```python
from build123d import *

# Parameters (mm, degrees)
F0_W     = 20
F0_H     = 20
F0_R     = 1.75
F0_R_2   = 1.1
F1_DEPTH = 3
F2_DEPTH = 1.4
F0_W_2   = 7.5
F3_DEPTH = 15
F4_DEPTH = 3
F5_W     = 3.5
F5_H     = 7.2
F6_DEPTH = 10
F7_R     = 2
F8_DEPTH = 25
F9_DEPTH = 7.5


with BuildPart() as f1:
    # F0 (on Right) → F1 (new body)
    with BuildSketch(Plane.YZ):
        Rectangle(F0_W, F0_H)
        with Locations((-5, -5)):
            Circle(F0_R, mode=Mode.SUBTRACT)
        with Locations((5, -5)):
            Circle(F0_R, mode=Mode.SUBTRACT)
        with Locations((-5, 5)):
            Circle(F0_R, mode=Mode.SUBTRACT)
        with Locations((5, 5)):
            Circle(F0_R, mode=Mode.SUBTRACT)
        with Locations((-5, 5)):
            Circle(F0_R)
        with Locations((-5, 5)):
            Circle(F0_R_2, mode=Mode.SUBTRACT)
        with Locations((5, 5)):
            Circle(F0_R)
        with Locations((5, 5)):
            Circle(F0_R_2, mode=Mode.SUBTRACT)
        with Locations((5, -5)):
            Circle(F0_R)
        with Locations((5, -5)):
            Circle(F0_R_2, mode=Mode.SUBTRACT)
        with Locations((-5, -5)):
            Circle(F0_R)
        with Locations((-5, -5)):
            Circle(F0_R_2, mode=Mode.SUBTRACT)
    extrude(amount=-F1_DEPTH)

    # F0 (on Right) → F2 (cut)
    with BuildSketch(Plane.YZ):
        with Locations((-5, 5)):
            Circle(F0_R)
        with Locations((-5, 5)):
            Circle(F0_R_2, mode=Mode.SUBTRACT)
        with Locations((5, 5)):
            Circle(F0_R)
        with Locations((5, 5)):
            Circle(F0_R_2, mode=Mode.SUBTRACT)
        with Locations((5, -5)):
            Circle(F0_R)
        with Locations((5, -5)):
            Circle(F0_R_2, mode=Mode.SUBTRACT)
        with Locations((-5, -5)):
            Circle(F0_R)
        with Locations((-5, -5)):
            Circle(F0_R_2, mode=Mode.SUBTRACT)
    extrude(amount=-F2_DEPTH, mode=Mode.SUBTRACT)

    # F9 (add, through all): a face of the model
    f9_faces = [f1.faces().sort_by_distance(p)[0] for p in [
        (-1.5, -10, 0),
    ]]


with BuildPart() as f3:
    # F0 (on Right) → F3 (new body)
    with BuildSketch(Plane.YZ):
        with Locations((-21.25, 0)):
            Rectangle(F0_W_2, F0_H)
    extrude(amount=F3_DEPTH)

    # F4 (add, through all): a face of the model
    f4_faces = [f3.faces().sort_by_distance(p)[0] for p in [
        (0, -21.25, 0),
    ]]
    extrude(f4_faces, amount=F4_DEPTH)

    # F5 (on face) → F6 (cut)
    with BuildSketch(Plane.YZ.offset(15)):
        with Locations((-21.25, 0)):
            Rectangle(F5_W, F5_H)
    extrude(amount=-F6_DEPTH, mode=Mode.SUBTRACT)

    # F7 (on face) → F8 (cut)
    with BuildSketch(Plane.XZ.offset(25)):
        with Locations((9.2, 0)):
            Circle(F7_R)
    extrude(amount=-F8_DEPTH, mode=Mode.SUBTRACT)


with BuildPart() as f1_1:
    add(f1.part)

    add(f3.part)  # F9 merges F3
    extrude(f9_faces, amount=F9_DEPTH)


solid = f1_1.part
```
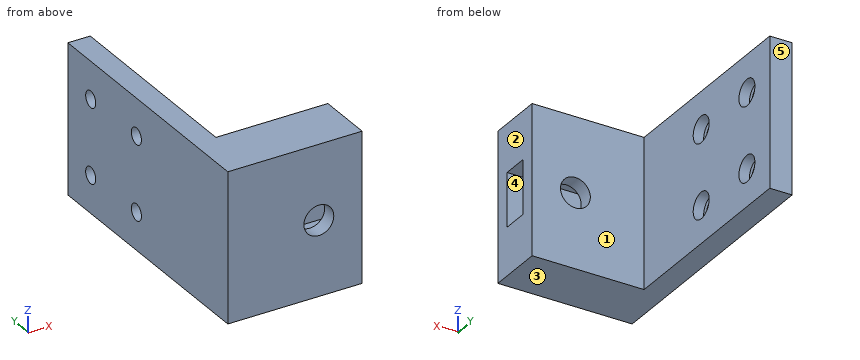
For this review, take the finished solid that the model builds, in its own axes (mm). Face numbers are marked on the shaded views. A direction names the side the tool comes from. Coordinates: 2 decimals unless noted, no trailing zeros. Loops run counter-clockwise (first coordinate to the right, second up) from the corner with the lowest first, then second, coordinate; pieces in that order, holes last. Notation, with made-up numbers: (31, 46) -> (44, 46) arc R29 cw to (44, 80) -> close; hole circle Ø5 at (14.5, 65). An arc over 180 degrees is marked (long way). Return JSON: item names as keys, results as strings. Group by question number.
(1) To check wall thickness, follow L1, parallel to Z at x = -0.85, y = -5; L2, parallel to Z at x = -1.75, y = -5; L3, parallel to Y at x = 6, z = 2.25. State the ranges of each line that lie inside material, in increasing order.
(2) Mouldability with a two-part tool opening along Z and no side actions: class the marked faces 3, 4 and 5 as pulls with the +Z half, pulls with the -Z half, needs draft (parallel to the pull), parting line crosses it, or undercut.
(3) Consider section C-C, the plane y = -5. Give the boundary of the cut face in (x, z).
(4) Consider section B-B, the plane z = -5. Give the boundary of the cut face in (x, y).
(5) Tool access review of the marked faces 1 and 2: name each direction out of +Z, -Z, +X, -X, +Y, -Y from which nothing blocks a thin tool from reaching the whole face with its end or side.
(6) Consider section A-A, the plane x = 12. Give the boundary of the cut face in (y, z), plus the area to 3 significant figures.
(7) Consider section D-D, the plane x = 9.2. Give the boundary of the cut face in (y, z), plus the area to 3 significant figures.
(8) For pin 1 Ø4.5 at (y, z) = (-5, 5) entering from +X; pin 2 Ø3 at (x, z) = (2, -2.5) entering from +Y; pin 3 Ø1.8 at (y, z) = (-21.5, 0) entering from +X, all flat-tipped, find the tip position at first contact; note any pin that passes through.
Results below:
{
 "1": {"L1": "z = -10 to -6.75, -3.25 to 3.25, 6.75 to 10", "L2": "z = -10 to -6.1, -3.9 to 3.9, 6.1 to 10", "L3": "y = -25 to -23, -19.5 to -17.5"},
 "2": {"face 3": "pulls with the -Z half", "face 4": "undercut", "face 5": "needs draft"},
 "3": {"outline": "(-3, -10) -> (0, -10) -> (0, -6.75) -> (-1.4, -6.75) -> (-1.4, -6.1) -> (-3, -6.1) -> close; (-3, -3.9) -> (-1.4, -3.9) -> (-1.4, -3.25) -> (0, -3.25) -> (0, 3.25) -> (-1.4, 3.25) -> (-1.4, 3.9) -> (-3, 3.9) -> close; (-3, 6.1) -> (-1.4, 6.1) -> (-1.4, 6.75) -> (0, 6.75) -> (0, 10) -> (-3, 10) -> close"},
 "4": {"outline": "(-3, -25) -> (15, -25) -> (15, -17.5) -> (0, -17.5) -> (0, -6.75) -> (-1.4, -6.75) -> (-1.4, -6.1) -> (-3, -6.1) -> close; (-3, -3.9) -> (-1.4, -3.9) -> (-1.4, -3.25) -> (0, -3.25) -> (0, 3.25) -> (-1.4, 3.25) -> (-1.4, 3.9) -> (-3, 3.9) -> close; (-3, 6.1) -> (-1.4, 6.1) -> (-1.4, 6.75) -> (0, 6.75) -> (0, 10) -> (-3, 10) -> close"},
 "5": {"face 1": "+Z, -Z, +X, +Y", "face 2": "+Z, -Z, +X, +Y, -Y"},
 "6": {"outline": "(-25, -10) -> (-17.5, -10) -> (-17.5, 10) -> (-25, 10) -> close; hole (-23, -3.6) -> (-19.5, -3.6) -> (-19.5, 3.6) -> (-23, 3.6) -> close", "area": "125 mm2"},
 "7": {"outline": "(-25, -10) -> (-17.5, -10) -> (-17.5, -2) -> (-19.5, -2) -> (-19.5, -3.6) -> (-23, -3.6) -> (-23, -2) -> (-25, -2) -> close; (-25, 2) -> (-23, 2) -> (-23, 3.6) -> (-19.5, 3.6) -> (-19.5, 2) -> (-17.5, 2) -> (-17.5, 10) -> (-25, 10) -> close", "area": "109 mm2"},
 "8": {"pin 1": "stops at x = 0", "pin 2": "stops at y = -17.5", "pin 3": "stops at x = 5"}
}
